Work out the finished part from the listing and answer in its coordinate system (mm). A direction names the side the tool comes from. Coordinates: 2 decimals unless noted, no trailing zeros. Order: outer loops, then holes, each group sorted by start corner. A loop starts at its lowest first (then second) coordinate and runs counter-clockwise, first axis right, second up. Notation, with made-up numbers: M 30,21.25 L 37,21.25 A30 cw 37,44.25 Z; hole C -39,5.25 d3. An arc over 180 degrees is marked long. Answer in a Markdown table with one row per item. Add a question column.
Item 1: The part is cut by section C-C (y = 7). Write down the section's boundary in (x, z).
Item 2: Flat-ended cylindrical pins translate along their axes: pin 1 Ø1.5 at (x, z) = (2, -112.5) entering from +Y; pin 2 Ø0.9 at (x, y) = (1, 11) entering from +Z. Find the tip coordinate at first contact, or state that the pin passes through.
Item 3: Which of the six approach directions +Z, -Z, +X, -X, +Y, -Y give full straight-line access (tool end or side, diameter ignored) to faces 1 (the face through (2, 13, -3)), 2 (the face through (1, 2, -111)), 3 (the face through (1, 24, -111)), 4 (the face through (1, 23, 0))?
Item 4: The part is cut by section B-B (y = 14). Write down the section's boundary in (x, z).
Item 5: The part is cut by section A-A (x = 1.5). Write down the section's boundary in (y, z).
Item 6: The mould has two halves that part along Y. Classify faces 5 (the face through (2, 21, -110)), 6 (the face through (1, 0, -55)), 7 (the face through (1, 3, 0)): released by +Y, released by -Y, zero draft, split by the parting line, or undercut.
Item 7: Consider line 1 (Z direction, x = 1.2, y = 21); line 2 (Z direction, x = 0.2, y = 24.5). Determine where each line is inside the solid, lowest interval first. Write a range as from..to.
from build123d import *

# Parameters (mm, degrees)
SKETCH_1_W          = 111
SKETCH_1_H          = 26
EXTRUDE_1_DEPTH     = 3
SKETCH_2_W          = 3
SKETCH_2_H          = 14
EXTRUDE_2_DEPTH     = 3
SKETCH_3_W          = 3
SKETCH_3_H          = 14
CUT_EXTRUDE_1_DEPTH = 5
SKETCH_4_R          = 1
CUT_EXTRUDE_2_DEPTH = 10


with BuildPart() as part:
    # 스케치1 → 보스-돌출1 (new body)
    with BuildSketch(Plane(origin=(0, 0, 0), x_dir=(0, 0, -1), z_dir=(1, 0, 0))):
        with Locations((55.5, 13)):
            Rectangle(SKETCH_1_W, SKETCH_1_H)
    extrude(amount=EXTRUDE_1_DEPTH)

    # 스케치2 → 보스-돌출2 (add)
    with BuildSketch(Plane(origin=(3, 0, 0), x_dir=(0, 0, -1), z_dir=(1, 0, 0))):
        with Locations((112.5, 13)):
            Rectangle(SKETCH_2_W, SKETCH_2_H)
    extrude(amount=-EXTRUDE_2_DEPTH)

    # 스케치3 → 컷-돌출1 (cut)
    with BuildSketch(Plane(origin=(3, 0, 0), x_dir=(0, 0, -1), z_dir=(1, 0, 0))):
        with Locations((1.5, 13)):
            Rectangle(SKETCH_3_W, SKETCH_3_H)
    extrude(amount=-CUT_EXTRUDE_1_DEPTH, mode=Mode.SUBTRACT)

    # 스케치4 → 컷-돌출2 (cut)
    with BuildSketch(Plane(origin=(3, 0, 0), x_dir=(0, 0, -1), z_dir=(1, 0, 0))):
        with Locations((111, 21)):
            Circle(SKETCH_4_R)
        with Locations((111, 5)):
            Circle(SKETCH_4_R)
        with Locations((3, 19)):
            Circle(SKETCH_4_R)
        with Locations((3, 7)):
            Circle(SKETCH_4_R)
    extrude(amount=-CUT_EXTRUDE_2_DEPTH, mode=Mode.SUBTRACT)


solid = part.part
Reply:
| question | item | result |
|---|---|---|
| 1 | outline | M 0,-114 L 3,-114 L 3,-4 L 0,-4 Z |
| 2 | pin 1 | stops at y = 20 |
| 2 | pin 2 | stops at z = -3 |
| 3 | face 1 | +Z, +X, -X |
| 3 | face 2 | -Z, +X, -X, -Y |
| 3 | face 3 | -Z, +X, -X, +Y |
| 3 | face 4 | +Z, +X, -X, +Y, -Y |
| 4 | outline | M 0,-114 L 3,-114 L 3,-3 L 0,-3 Z |
| 5 | outline | M 0,-111 L 4,-111 A1 cw 6,-111 L 6,-114 L 20,-114 L 20,-111 A1 cw 22,-111 L 26,-111 L 26,0 L 20,0 L 20,-3 A1 cw 18,-3 L 8,-3 A1 cw 6,-3 L 6,0 L 0,0 Z |
| 6 | face 5 | undercut |
| 6 | face 6 | released by -Y |
| 6 | face 7 | zero draft |
| 7 | line 1 | z = -110..0 |
| 7 | line 2 | z = -111..0 |
